Read the model definition and answer for the solid it produces. Units are mm, in the model's axes. Give positions to 0.01 mm unless a question says otherwise; leave off trailing zeros. Write each loop counter-clockwise with the first axis right and the second up, starting at its lowest first coordinate (ties: lowest second). Pieces come first, ordered by that corner, then holes. Notation, with made-up numbers: (22.25, 81) -> (56.25, 81) arc R9 cw to (56.25, 90) -> close; hole circle Ø10 at (-13.75, 4.25). An arc over 180 degrees is marked (long way). Use a Markdown table: item, result.
from build123d import *

# Parameters (mm, degrees)
SKETCH2_R           = 0.85
BOSS_EXTRUDE1_DEPTH = 0.75
FILLET1_R           = 7.400617123
FILLET2_R           = 1.850154281


with BuildPart() as part:
    # Sketch2 → Boss-Extrude1 (new body, symmetric)
    with BuildSketch(Plane.XY):
        with BuildLine():
            Line((-5.084030917, -7.311581435), (-5.231445397, -3.68673013))
            ThreePointArc((-5.231445397, -3.68673013), (-6.08432946, 3.458247986), (0, 7.3))
            Line((0, 7.3), (0, 5.5))
            ThreePointArc((0, 5.5), (-5.499162323, 0.095988235), (-0.191947232, -5.496649549))
            Line((-0.191947232, -5.496649549), (-0.310794848, -8.9))
            ThreePointArc((-0.310794848, -8.9), (-2.811904096, -8.449839572), (-5.084030917, -7.311581435))
        make_face()
        with Locations((-2.274269541, -6.834234779)):
            Circle(SKETCH2_R, mode=Mode.SUBTRACT)
    extrude(amount=BOSS_EXTRUDE1_DEPTH, both=True)

    # Fillet1
    fillet1_edges = [part.edges().sort_by_distance(p)[0] for p in [
        (-5.231445397, -3.68673013, 0),
    ]]
    fillet(fillet1_edges, radius=FILLET1_R)

    # Fillet2
    fillet2_edges = [part.edges().sort_by_distance(p)[0] for p in [
        (-5.084030917, -7.311581435, 0),
    ]]
    fillet(fillet2_edges, radius=FILLET2_R)

    # Mirror1: part across plane


with BuildPart() as part_1:
    add(part.part)
    add(part.part.mirror(Plane(origin=(0, 7.3, 0.75), x_dir=(0, 0, 1), z_dir=(-1, 0, 0))))


solid = part_1.part
Item 1: A cutting plane is placed at A-A (y = -0.75). Give the vertices of the cut face in (x, z).
Return value:
| item | result |
|---|---|
| outline | (-6.61, -0.75) -> (-5.45, -0.75) -> (-5.45, 0.75) -> (-6.61, 0.75) -> close; (5.45, -0.75) -> (6.61, -0.75) -> (6.61, 0.75) -> (5.45, 0.75) -> close |
Item 2: This flat-tipped pin is pushed along its axis until it touches: P1, Ø3, axis at x = -3, y = 1.5, coming from the -Z side. Where does it stop, or does it pass through?
Return value:
| item | result |
|---|---|
| P1 | through |
Item 3: A cutting plane is placed at C-C (z = 0.2). Give the vertices of the cut face in (x, y).
Return value:
| item | result |
|---|---|
| outline | (-5.98, -2.55) arc R7.4 cw to (-5.15, -5.66) -> (-5.12, -6.32) arc R1.85 ccw to (-4.13, -7.89) arc R8.91 ccw to (-0.31, -8.9) -> (-0.19, -5.5) arc R5.5 cw (long way) to (0.19, -5.5) -> (0.31, -8.9) arc R8.91 ccw to (4.13, -7.89) arc R1.85 ccw to (5.12, -6.32) -> (5.15, -5.66) arc R7.4 cw to (5.98, -2.55) arc R6.74 ccw (long way) to start; hole circle Ø1.7 at (-2.27, -6.83); hole circle Ø1.7 at (2.27, -6.83) |
Item 4: For a pull along Z with two mould halves and no side action, classify faces 1 (the face through (-1, -6, -0.75)), 2 (the face through (-1, -6, 0.75)), 3 (the face through (4.846, -7.227, 0.01)) as +Z half, -Z half, draft (parallel to the pull), parting line (faces both ways), or undercut.
Return value:
| item | result |
|---|---|
| face 1 | -Z half |
| face 2 | +Z half |
| face 3 | draft |
Item 5: A cutting plane is placed at B-B (x = -4.5). Give the vertices of the cut face in (y, z), then the cut area to 3 significant figures.
Return value:
| item | result |
|---|---|
| outline | (-7.64, -0.75) -> (-3.16, -0.75) -> (-3.16, 0.75) -> (-7.64, 0.75) -> close; (3.16, -0.75) -> (5.58, -0.75) -> (5.58, 0.75) -> (3.16, 0.75) -> close |
| area | 10.3 mm^2 |
Item 6: A cutting plane is placed at D-D (x = -2.25). Give the vertices of the cut face in (y, z).
Return value:
| item | result |
|---|---|
| outline | (-8.62, -0.75) -> (-7.68, -0.75) -> (-7.68, 0.75) -> (-8.62, 0.75) -> close; (-5.98, -0.75) -> (-5.02, -0.75) -> (-5.02, 0.75) -> (-5.98, 0.75) -> close; (5.02, -0.75) -> (6.91, -0.75) -> (6.91, 0.75) -> (5.02, 0.75) -> close |
Item 7: Straight lines are drawn through the part: line 1 along Y through (x, z) = (-3, -0.65); line 2 along X through (y, z) = (-6.75, 0.1); line 3 along Y through (x, z) = (0, -0.55). For each, find the intervals that lie inside material, in ascending order. Write a range as [from, to].
Return value:
| item | result |
|---|---|
| line 1 | [-8.38, -7.28], [-6.39, -4.61], [4.61, 6.6] |
| line 2 | [-5.06, -3.12], [-1.43, -0.24], [0.24, 1.43], [3.12, 5.06] |
| line 3 | [5.5, 7.3] |
